from build123d import *

# Parameters (mm, degrees)
SKETCH_1_R          = 10
EXTRUDE_1_DEPTH     = 35
SKETCH_2_W          = 40
SKETCH_2_H          = 24
EXTRUDE_2_DEPTH     = 10
EXTRUDE_3_DEPTH     = 8
EXTRUDE_4_DEPTH     = 8
SKETCH_5_R          = 5
CUT_EXTRUDE_1_DEPTH = 76
SKETCH_6_R          = 3.4
CUT_EXTRUDE_2_DEPTH = 20


with BuildPart() as part:
    # 草图1 → 凸台-拉伸1 (new body)
    with BuildSketch(Plane(origin=(0, 0, 0), x_dir=(1, 0, 0), z_dir=(0, 1, 0))):
        with Locations(Location((0, 0, 0), (0, 0, 270))):
            Circle(SKETCH_1_R)
    extrude(amount=EXTRUDE_1_DEPTH)

    # 草图2 → 凸台-拉伸2 (add)
    with BuildSketch(Plane(origin=(0, 35, 0), x_dir=(1, 0, 0), z_dir=(0, 1, 0))):
        Rectangle(SKETCH_2_W, SKETCH_2_H)
    extrude(amount=EXTRUDE_2_DEPTH)

    # 草图3 → 凸台-拉伸3 (add)
    with BuildSketch(Plane(origin=(12, 0, 0), x_dir=(0, 0, -1), z_dir=(1, 0, 0))):
        with BuildLine():
            Line((12, 45), (12, 63))
            ThreePointArc((12, 63), (0, 75), (-12, 63))
            Line((-12, 63), (-12, 45))
            Line((-12, 45), (12, 45))
        make_face()
    extrude(amount=EXTRUDE_3_DEPTH)

    # 草图4 → 凸台-拉伸4 (add)
    with BuildSketch(Plane(origin=(-20, 0, 0), x_dir=(0, 0, -1), z_dir=(1, 0, 0))):
        with BuildLine():
            Line((12, 45), (12, 63))
            ThreePointArc((12, 63), (0, 75), (-12, 63))
            Line((-12, 63), (-12, 45))
            Line((-12, 45), (12, 45))
        make_face()
    extrude(amount=EXTRUDE_4_DEPTH)

    # 草图5 → 切除-拉伸1 (cut, symmetric)
    with BuildSketch(Plane(origin=(-20, 0, 0), x_dir=(0, 0, -1), z_dir=(1, 0, 0))):
        with Locations((0, 63)):
            Circle(SKETCH_5_R)
    extrude(amount=CUT_EXTRUDE_1_DEPTH, both=True, mode=Mode.SUBTRACT)

    # 草图6 → 切除-拉伸2 (cut)
    with BuildSketch(Plane(origin=(0, 0, 0), x_dir=(1, 0, 0), z_dir=(0, 1, 0))):
        with Locations(Location((0, 0, 0), (0, 0, 270))):
            Circle(SKETCH_6_R)
    extrude(amount=CUT_EXTRUDE_2_DEPTH, mode=Mode.SUBTRACT)


solid = part.part
Build history of the part. All positions in model axes, mm. A direction names the side the tool comes from. Round coordinates to 2 decimals unless told otherwise and drop trailing zeros. Loops run counter-clockwise (first coordinate to the right, second up) from the corner with the lowest first, then second, coordinate; pieces in that order, holes last. Notation, with made-up numbers: (42, 9.5) -> (75, 9.5) arc R20 ccw to (75, 27.5) -> close; hole circle Ø5 at (-35, -2). An arc over 180 degrees is marked (long way). Answer in a Markdown table with one row per item.
Item 1: Saw through at A-A (z = 0). Write the cut outline in (x, y).
Answers below:
| item | result |
|---|---|
| outline | (-20, 35) -> (-10, 35) -> (-10, 0) -> (-3.4, 0) -> (-3.4, 20) -> (3.4, 20) -> (3.4, 0) -> (10, 0) -> (10, 35) -> (20, 35) -> (20, 58) -> (12, 58) -> (12, 45) -> (-12, 45) -> (-12, 58) -> (-20, 58) -> close; (-20, 68) -> (-12, 68) -> (-12, 75) -> (-20, 75) -> close; (12, 68) -> (20, 68) -> (20, 75) -> (12, 75) -> close |
Item 2: Which spindle directions (+Z, -Z, +X, -X, +Y, -Y) get a long thin tool onto all of the face, cutting with end or side? Do faces 1 (the cylindrical face through (16, 67, -3)), 2 (the flat face through (9, 35, -6)), 3 (the flat face through (-12, 57, 0)). Say none if no direction does.
Answers below:
| item | result |
|---|---|
| face 1 | +X, -X |
| face 2 | -Y |
| face 3 | +Z, -Z, +Y |
Item 3: Saw through at C-C (y = 64.5). Write the cut outline in (x, z), and give its area (3 significant figures).
Answers below:
| item | result |
|---|---|
| outline | (-20, -11.91) -> (-12, -11.91) -> (-12, -4.77) -> (-20, -4.77) -> close; (-20, 4.77) -> (-12, 4.77) -> (-12, 11.91) -> (-20, 11.91) -> close; (12, -11.91) -> (20, -11.91) -> (20, -4.77) -> (12, -4.77) -> close; (12, 4.77) -> (20, 4.77) -> (20, 11.91) -> (12, 11.91) -> close |
| area | 228 mm² |
Item 4: Pin check, flat tips, straight feed: pin 1 (12 mm diameter, centred on x = 14.5, y = 26, fed in from -Z); pin 2 (7 mm diameter, centred on x = 3.5, z = -4, fed in from +Y); pin 3 (1.5 mm diameter, centred on x = -12, y = 30, fed in from +Z); pin 4 (3 mm diameter, centred on x = -9, y = 8, fed in from +Z). Stop position of each tip, or through.
Answers below:
| item | result |
|---|---|
| pin 1 | stops at z = -5.27 |
| pin 2 | stops at y = 45 |
| pin 3 | passes through |
| pin 4 | stops at z = 6.61 |
Item 5: Saw through at D-D (x = 0). Write the cut outline in (y, z), and give its area (3 significant figures).
Answers below:
| item | result |
|---|---|
| outline | (0, -10) -> (35, -10) -> (35, -12) -> (45, -12) -> (45, 12) -> (35, 12) -> (35, 10) -> (0, 10) -> (0, 3.4) -> (20, 3.4) -> (20, -3.4) -> (0, -3.4) -> close |
| area | 804 mm² |
Item 6: Drill centre lines: L1, parallel to X at y = 5.5, z = 0; L2, parallel to X at y = 68.5, z = -7.25; L3, parallel to Z at x = 1, y = 18. Where is each one in solid material? Low to high. Write a range as [from, to].
Answers below:
| item | result |
|---|---|
| L1 | x = [-10, -3.4], [3.4, 10] |
| L2 | x = [-20, -12], [12, 20] |
| L3 | z = [-9.95, -3.25], [3.25, 9.95] |
Item 7: Mould opens along Z. For faces 4 (the cylindrical face through (-16, 67, -3)), 5 (the flat face through (0, 43, -12)), 6 (the flat face through (0, 45, 0)), 7 (the cylindrical face through (16, 75, 0)) say: +Z half, -Z half, draft (parallel to the pull), parting line (faces both ways), or undercut.
Answers below:
| item | result |
|---|---|
| face 4 | undercut |
| face 5 | -Z half |
| face 6 | draft |
| face 7 | parting line |
Item 8: Saw through at B-B (x = -15). Write the cut outline in (y, z), and give its area (3 significant figures).
Answers below:
| item | result |
|---|---|
| outline | (35, -12) -> (63, -12) arc R12 ccw to (63, 12) -> (35, 12) -> close; hole circle Ø10 at (63, 0) |
| area | 820 mm² |
